Design review of the part shown in the three views and the two pictorial views. Dimensions are in mm from the part's minimum x, y and z. Give positions to 0.01 mm unless a question says otherwise; leave off trailing zeros. Loops run counter-clockwise (first coordinate to the right, second up) from the corner with the lowest first, then second, coordinate; pieces in that order, holes last.
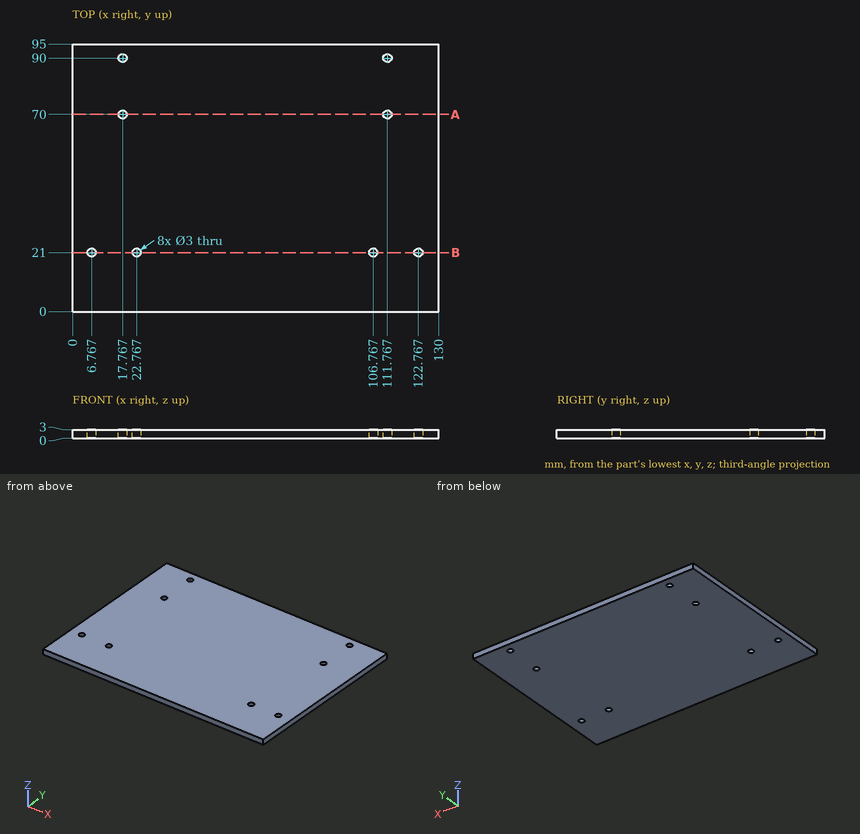
Q1. For probe 1 along X at (y, z) = (90, 2); probe 2 along Y at (x, z) = (122.5, 1.05); probe 3 along X at (y, z) = (91, 1.05) (1 decimal), list the stretches that pass through material, from the lowest coordinate up.
Answers:
probe 1: x = 0 to 16.27, 19.27 to 110.27, 113.27 to 130
probe 2: y = 0 to 19.52, 22.48 to 95
probe 3: x = 0 to 16.6, 18.9 to 110.6, 112.9 to 130
Q2. Consider section A-A on y = 70. Give the boundary of the cut face in (x, z).
Answers:
outline: (0, 0) - (16.27, 0) - (16.27, 3) - (0, 3) - close; (19.27, 0) - (110.27, 0) - (110.27, 3) - (19.27, 3) - close; (113.27, 0) - (130, 0) - (130, 3) - (113.27, 3) - close
Q3. Consider section B-B on y = 21. Give the boundary of the cut face in (x, z).
Answers:
outline: (0, 0) - (5.27, 0) - (5.27, 3) - (0, 3) - close; (8.27, 0) - (21.27, 0) - (21.27, 3) - (8.27, 3) - close; (24.27, 0) - (105.27, 0) - (105.27, 3) - (24.27, 3) - close; (108.27, 0) - (121.27, 0) - (121.27, 3) - (108.27, 3) - close; (124.27, 0) - (130, 0) - (130, 3) - (124.27, 3) - close
Q4. For pin 1 Ø5 at (x, y) = (22.77, 21) entering from +Z; pin 2 Ø1.8 at (x, y) = (17.77, 90) entering from -Z, all flat-tipped, find the tip position at first contact; note any pin that passes through.
Answers:
pin 1: stops at z = 3
pin 2: passes through
